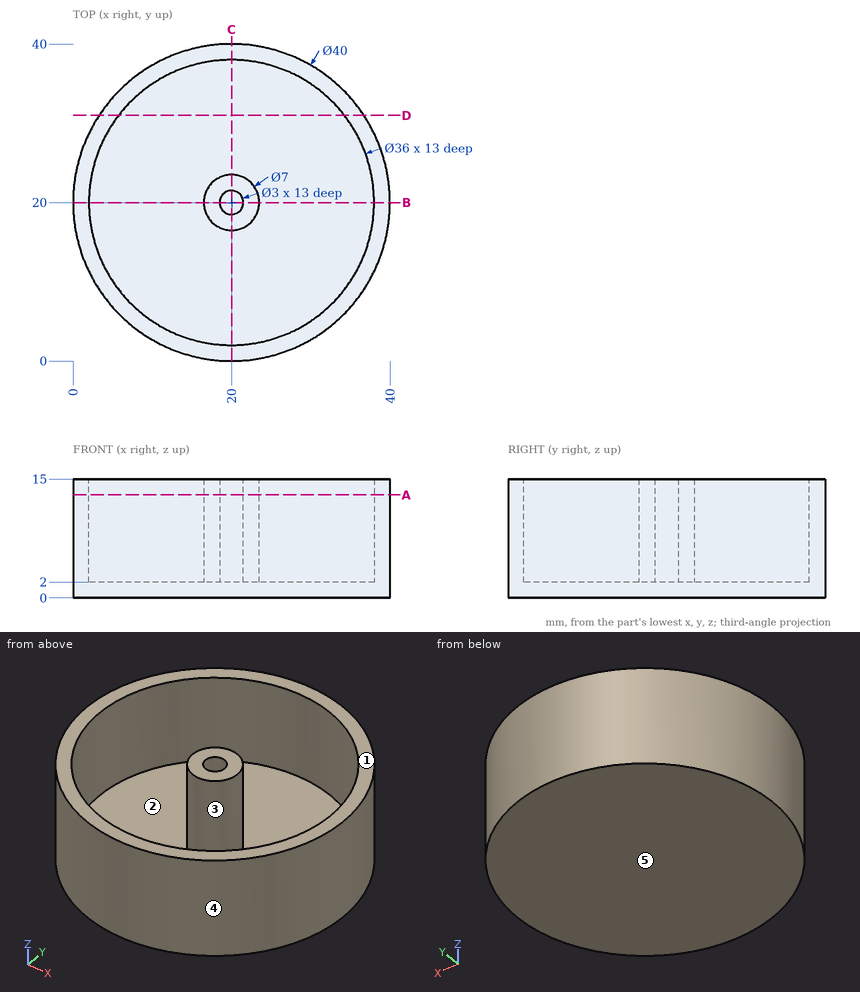
Geometry check sheet. Reference: drawing and pictorial views, mm from the part's lowest x, y, z. A direction names the side the tool comes from. Give positions to 0.01 mm unless a question says otherwise; leave off trailing zeros. Write each loop counter-clockwise with the first axis right and the second up, starting at its lowest first coordinate (ties: lowest second). Pieces come first, ordered by that corner, then holes. Notation, with made-up numbers: (78, 55) -> (99, 55) arc R36 ccw to (99, 92) -> close; hole circle Ø7 at (16.5, 80). An arc over 180 degrees is marked (long way). One line per item, written item: value. Start each with the question number.
Item 1: Tool access check on the marked faces 1 and 2. Record the directions out of +Z, -Z, +X, -X, +Y, -Y that give a thin tool (end or side, any length) a straight path to the whole face; none if there is none.
Item 2: Section check A-A on z = 13. Record the cut outline in (x, y).
Item 3: Section check D-D on y = 31. Record the cut outline in (x, z).
Item 4: Material ranges on probe 1 along Y at (x, z) = (20, 8.25); probe 2 along X at (y, z) = (21, 12); probe 3 along X at (y, z) = (23, 13.5), recorded low to high. Write a range as from..to.
Item 5: Draft check along X on the marked faces 3, 4 and 5. Enter one of: +X half, -X half, draft (parallel to the pull), parting line (faces both ways), or undercut.
Item 6: Section check B-B on y = 20. Record the cut outline in (x, z).
Item 7: Gauge pin test, flat ends, axial feed: pin 1 (1.5 mm diameter, centred on x = 19.5, y = 20.5, fed in from +Z); pin 2 (1 mm diameter, centred on x = 16, y = 12, fed in from -Z); pin 3 (1.5 mm diameter, centred on y = 29, z = 2, fed in from -X); pin 4 (1.5 mm diameter, centred on y = 28.5, z = 12, fed in from +X). Record the tip position at first contact, or that the pin passes through.
Results list:
1. face 1: +Z, +X, -X, +Y, -Y
1. face 2: +Z
2. outline: circle Ø40 at (20, 20); circle Ø7 at (20, 20); hole circle Ø36 at (20, 20); hole circle Ø3 at (20, 20)
3. outline: (3.3, 0) -> (36.7, 0) -> (36.7, 15) -> (34.25, 15) -> (34.25, 2) -> (5.75, 2) -> (5.75, 15) -> (3.3, 15) -> close
4. probe 1: 0..2, 16.5..18.5, 21.5..23.5, 38..40
4. probe 2: 0.03..2.03, 16.65..18.88, 21.12..23.35, 37.97..39.97
4. probe 3: 0.23..2.25, 18.2..21.8, 37.75..39.77
5. face 3: undercut
5. face 4: parting line
5. face 5: draft
6. outline: (0, 0) -> (40, 0) -> (40, 15) -> (38, 15) -> (38, 2) -> (23.5, 2) -> (23.5, 15) -> (21.5, 15) -> (21.5, 2) -> (18.5, 2) -> (18.5, 15) -> (16.5, 15) -> (16.5, 2) -> (2, 2) -> (2, 15) -> (0, 15) -> close
7. pin 1: z = 2
7. pin 2: z = 0
7. pin 3: x = 1.78
7. pin 4: x = 38.44
